Verification items for this drawing (mm, ordinates from the low corner). Coordinates: 2 decimals unless noted, no trailing zeros. Order: outer loops, then holes, each group sorted by start corner. A loop starts at its lowest first (then second) coordinate and runs counter-clockwise, first axis right, second up. Notation, with made-up numbers: M -22,14 L 14,14 A35 ccw 14,47 Z; hole C 58.5,-4 d1. An arc over 180 degrees is marked long. One line per item, written item: value. Start each with the question number.
1) Sectioned sample at B-B, the plane x = 4.5. Enter the section's corners in (y, z), then the cut area to 3 significant figures.
2) Sectioned sample at C-C, the plane x = 0.55. Enter the section's corners in (y, z), then the cut area to 3 significant figures.
3) Thickness scan on L1, parallel to X at y = 3.5, z = 28.5 (1 decimal); L2, parallel to Y at x = 3.55, z = 4; L3, parallel to X at y = 3, z = 29. Record the ranges inside material, lowest first. Write a range as from..to.
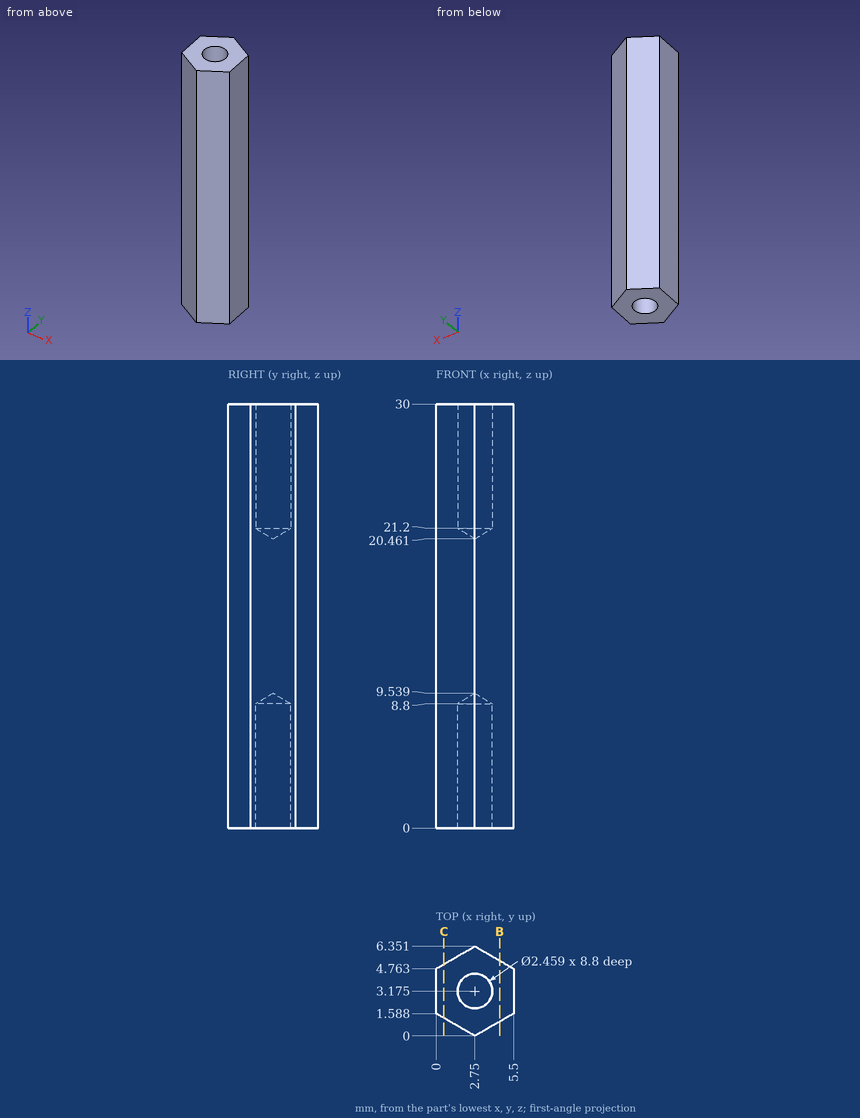
Final values:
1. outline: M 1.01,0 L 5.34,0 L 5.34,30 L 1.01,30 Z
1. area: 130 mm^2
2. outline: M 1.27,0 L 5.08,0 L 5.08,30 L 1.27,30 Z
2. area: 114 mm^2
3. L1: x = 0..1.6, 3.9..5.5
3. L2: y = 0.46..2.24, 4.11..5.89
3. L3: x = 0..1.53, 3.97..5.5
